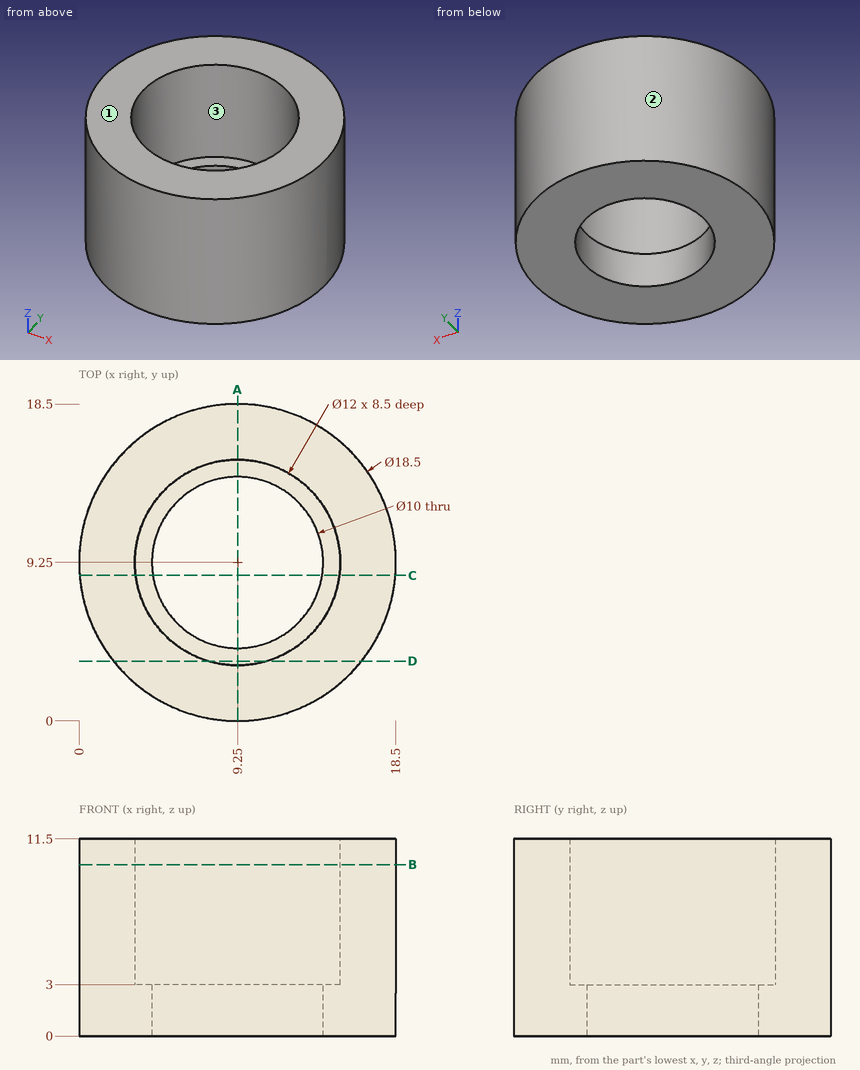
For this review, use the dimensioned drawing (mm, ordinates from the lowest corner) and the shaded views. Coordinates: 2 decimals unless noted, no trailing zeros. Order: outer loops, then holes, each group sorted by start corner. A loop starts at its lowest first (then second) coordinate and runs counter-clockwise, first axis right, second up. Notation, with made-up numbers: (-23, 79.25) -> (2, 79.25) arc R27 cw to (2, 97.25) -> close; hole circle Ø10 at (18.25, -40). An arc over 180 degrees is marked (long way). One line per item, written item: value. Start each with the question number.
Q1. For probe 1 along Y at (x, z) = (9.25, 6.5); probe 2 along X at (y, z) = (7.75, 9.5), list the stretches that pass through material, from the lowest coordinate up.
Q2. Take a section at A-A, the plane x = 9.25. State the section outline as (y, z) points.
Q3. Take a section at B-B, the plane z = 10. State the section outline as (x, y) points, then the cut area to 3 significant figures.
Q4. Insertion check: pin 1 Ø4 at (y, z) = (11.5, 3.5) entering from +X; pin 2 Ø3 at (y, z) = (13.5, 4) entering from -X; pin 3 Ø4 at (x, z) = (12.5, 7) entering from -Y. Each pin has a flat end and moves straight along its axis. Give the tip position at first contact, or say it passes through.
Q5. Take a section at C-C, the plane y = 8.5. State the section outline as (x, z) points, then the cut area to 3 significant figures.
Q6. Mouldability with a two-part tool opening along Y and no side actions: class the marked faces 1, 2 and 3 as pulls with the +Y half, pulls with the -Y half, needs draft (parallel to the pull), parting line crosses it, or undercut.
Q7. Take a section at D-D, the plane y = 3.5. State the section outline as (x, z) points, then the cut area to 3 significant figures.
Values follow:
1. probe 1: y = 0 to 3.25, 15.25 to 18.5
1. probe 2: x = 0.12 to 3.44, 15.06 to 18.38
2. outline: (0, 0) -> (4.25, 0) -> (4.25, 3) -> (3.25, 3) -> (3.25, 11.5) -> (0, 11.5) -> close; (14.25, 0) -> (18.5, 0) -> (18.5, 11.5) -> (15.25, 11.5) -> (15.25, 3) -> (14.25, 3) -> close
3. outline: circle Ø18.5 at (9.25, 9.25); hole circle Ø12 at (9.25, 9.25)
3. area: 156 mm2
4. pin 1: stops at x = 18.5
4. pin 2: stops at x = 0.42
4. pin 3: stops at y = 0.08
5. outline: (0.03, 0) -> (4.31, 0) -> (4.31, 3) -> (3.3, 3) -> (3.3, 11.5) -> (0.03, 11.5) -> close; (14.19, 0) -> (18.47, 0) -> (18.47, 11.5) -> (15.2, 11.5) -> (15.2, 3) -> (14.19, 3) -> close
5. area: 81.2 mm2
6. face 1: needs draft
6. face 2: parting line crosses it
6. face 3: undercut
7. outline: (2, 0) -> (16.5, 0) -> (16.5, 11.5) -> (10.96, 11.5) -> (10.96, 3) -> (7.54, 3) -> (7.54, 11.5) -> (2, 11.5) -> close
7. area: 138 mm2
